Autodesk Inventor part; units mm, degrees
ref_plane "paddle_to_bracket_XY" through (0, -1.3716, 0) normal (0, 0, -1) x (1, 0, 0)
ref_plane "paddle_to_bracket_YZ" through (0, -1.3716, 0) normal (1, 0, 0) x (0, -1, 0)
ref_plane "paddle_to_bracket_ZX" through (0, -1.3716, 0) normal (0, -1, 0) x (0, 0, -1)
sketch "Sketch_1" plane through (0, 0, 0) normal (1, 0, 0) x (0, 1, 0)
  line L0 (-1.27, 0) -> (13.4366, 0)
  line L1 (13.4366, 0) -> (13.4366, -1.2446)
  line L2 (13.4366, -1.2446) -> (14.7066, -1.2446)
  line L3 (14.7066, -1.2446) -> (14.7066, -2.1427)
  line L4 (14.7066, -2.1427) -> (14.3474, -2.5019)
  line L5 (14.3474, -2.5019) -> (2.54, -2.5019)
  line L6 (2.54, -2.5019) -> (2.54, -1.4859)
  line L7 (2.54, -1.4859) -> (-1.27, -1.4859)
  line L8 (-1.27, -1.4859) -> (-1.27, 0)
  line L9 (-1.27, 0) -> (13.4366, 0)
revolve "Revolution1" add sketch "Sketch_1" angle 360 about axis through (0, -1.27, 0) along (0, -1, 0)
ref_plane "paddle_to_bracket_XY" through (0, -1.3716, 0) normal (0, 0, -1) x (1, 0, 0)
ref_plane "paddle_to_bracket_YZ" through (0, -1.3716, 0) normal (1, 0, 0) x (0, -1, 0)
ref_plane "paddle_to_bracket_ZX" through (0, -1.3716, 0) normal (0, -1, 0) x (0, 0, -1)
ref_plane "paddle_to_led_XY" through (0, 13.8525, 0) normal (0, 1, 0) x (1, 0, 0)
ref_plane "paddle_to_led_YZ" through (0, 13.8525, 0) normal (1, 0, 0) x (0, 0, -1)
ref_plane "paddle_to_led_ZX" through (0, 13.8525, 0) normal (0, 0, -1) x (0, 1, 0)
ref_plane "paddle_to_led_green_XY" through (0, 13.8525, 0) normal (0, 1, 0) x (1, 0, 0)
ref_plane "paddle_to_led_green_YZ" through (0, 13.8525, 0) normal (1, 0, 0) x (0, 0, -1)
ref_plane "paddle_to_led_green_ZX" through (0, 13.8525, 0) normal (0, 0, -1) x (0, 1, 0)
ref_plane "rocker_to_bracket_XY" through (0, 1.778, 0) normal (0, -1, 0) x (1, 0, 0)
ref_plane "rocker_to_bracket_YZ" through (0, 1.778, 0) normal (1, 0, 0) x (0, 0, 1)
ref_plane "rocker_to_bracket_ZX" through (0, 1.778, 0) normal (0, 0, 1) x (0, -1, 0)
ref_plane "toggle_to_bc_XY" through (0, 0, 0) normal (0, 1, 0) x (1, 0, 0)
ref_plane "toggle_to_bc_YZ" through (0, 0, 0) normal (1, 0, 0) x (0, 0, -1)
ref_plane "toggle_to_bc_ZX" through (0, 0, 0) normal (0, 0, -1) x (0, 1, 0)
ref_plane "toggle_to_led_XY" through (0, 13.4366, 0) normal (0, 1, 0) x (1, 0, 0)
ref_plane "toggle_to_led_YZ" through (0, 13.4366, 0) normal (1, 0, 0) x (0, 0, -1)
ref_plane "toggle_to_led_ZX" through (0, 13.4366, 0) normal (0, 0, -1) x (0, 1, 0)
ref_plane "toggle_to_led_green_XY" through (0, 13.4366, 0) normal (0, 1, 0) x (1, 0, 0)
ref_plane "toggle_to_led_green_YZ" through (0, 13.4366, 0) normal (1, 0, 0) x (0, 0, -1)
ref_plane "toggle_to_led_green_ZX" through (0, 13.4366, 0) normal (0, 0, -1) x (0, 1, 0)
properties part number "M211L01W-actuator"
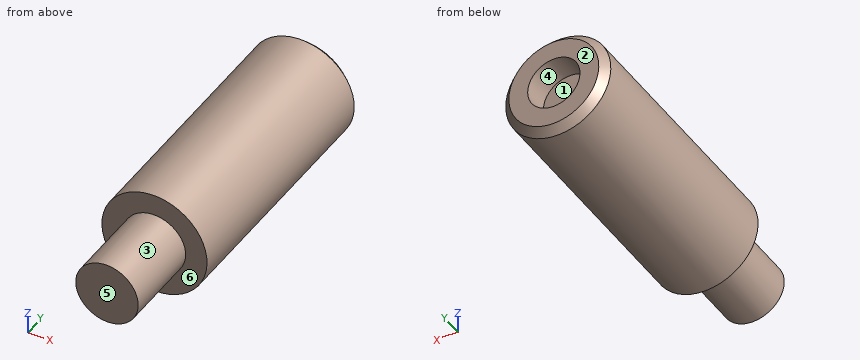
CAD build for the part. Positions are in the model's coordinates, mm. Face numbers are marked on the shaded views. A direction names the side the tool comes from. Coordinates: 2 decimals unless noted, no trailing zeros. Loops run counter-clockwise (first coordinate to the right, second up) from the corner with the lowest first, then second, coordinate; pieces in that order, holes last. Notation, with made-up numbers: (26.5, 36.25) -> (79.5, 36.25) arc R22 cw to (79.5, 61.25) -> close; hole circle Ø7 at (-14, 74). An arc over 180 degrees is marked (long way). One line per item, written item: value.
1. Slice it at C-C on y = 3.5. Write the cut outline in (x, z), and give its area (3 significant figures).
Answers:
outline: circle Ø5 at (0, 0)
area: 19.7 mm^2
2. Which spindle directions (+Z, -Z, +X, -X, +Y, -Y) get a long thin tool onto all of the face, cutting with end or side? Do the marked faces 4, 5 and 6. Say none if no direction does.
Answers:
face 4: +Y
face 5: +Z, -Z, +X, -X, -Y
face 6: -Y
3. Flat gauge pin, fed straight in: P1, Ø1.5, axis at x = 0.5, y = 1.5, coming from the -Z side. Where does the tip first touch, or does it go through?
Answers:
P1: stops at z = -1.49
4. Drill centre lines: line 1 (X direction, y = 14.05, z = 0); line 2 (Y direction, x = 0.2, z = 0.2); line 3 (Y direction, x = 0.85, z = 1.8). Where is each one in solid material? Low to high. Write a range as [from, to].
Answers:
line 1: x = [-2.5, -1.24], [1.24, 2.5]
line 2: y = [-1.27, 13.44]
line 3: y = [2.54, 14.71]
5. Pull direction Z, two halves, no side cores. Call the marked faces 1, 2 and 3: pulls with the +Z half, pulls with the -Z half, needs draft (parallel to the pull), parting line crosses it, or undercut.
Answers:
face 1: undercut
face 2: needs draft
face 3: parting line crosses it
6. Slice it at B-B on x = 0. Write the cut outline in (y, z), and give its area (3 significant figures).
Answers:
outline: (-1.27, -1.49) -> (2.54, -1.49) -> (2.54, -2.5) -> (14.35, -2.5) -> (14.71, -2.14) -> (14.71, -1.24) -> (13.44, -1.24) -> (13.44, 1.24) -> (14.71, 1.24) -> (14.71, 2.14) -> (14.35, 2.5) -> (2.54, 2.5) -> (2.54, 1.49) -> (-1.27, 1.49) -> close
area: 68.9 mm^2
7. Slice it at A-A on z = 0. Write the cut outline in (x, y).
Answers:
outline: (-2.5, 2.54) -> (-1.49, 2.54) -> (-1.49, -1.27) -> (1.49, -1.27) -> (1.49, 2.54) -> (2.5, 2.54) -> (2.5, 14.35) -> (2.14, 14.71) -> (1.24, 14.71) -> (1.24, 13.44) -> (-1.24, 13.44) -> (-1.24, 14.71) -> (-2.14, 14.71) -> (-2.5, 14.35) -> close
